For this review, take the finished solid that the model builds, in its own axes (mm). A direction names the side the tool comes from. Give positions to 0.01 mm unless a question says otherwise; leave off trailing zeros. Order: outer loops, then holes, each group sorted by start corner. A loop starts at its lowest first (then second) coordinate and runs counter-clockwise, first axis right, second up. Notation, with made-up numbers: M -26,45 L -15,45 A19 ccw -15,52 Z; hole C 28,-4 d8. An arc over 180 degrees is marked long. Use CSV: the item, a comma, the result in double quotes. Start each with the question number.
(1) Clearance check with flat-ended pins moving along their axes: P1, Ø4, axis at x = 32, y = -44.5, coming from the -Z side; P2, Ø1.2, axis at y = 33, z = 2, coming from the +X side. State where each tip first meets the part, or that it passes through.
(2) Consider section C-C (x = 31). Write out the cut boundary in (y, z).
(3) Draft analysis for pull direction X (two halves, no side actions). For faces 1 (the face through (60, -60, 2)), 2 (the face through (0.752, 39.287, 1.972)), 3 (the face through (11.4, 32.19, 1.97)), state which applies: pulls with the +X half, pulls with the -X half, needs draft (parallel to the pull), parting line crosses it, or undercut.
(4) Consider section D-D (z = 1.25). Give the number of separate pieces and of enclosed holes in the cut face, and give its area (3 significant figures).
(5) Consider section B-B (y = 10). Write out the cut boundary in (x, z), and give its area (3 significant figures).
(6) Wall thickness on L1, parallel to Y at x = 70, z = 2.75; L2, parallel to Y at x = 50.5, z = 1.15; L3, parallel to Y at x = 30, z = 2: over which ranges is each line inside the solid? List them lowest first. Write a range as from..to.
(7) Tool access review of faces 4 (the face through (60, 0, 2)), 5 (the face through (9.44, 7.46, 1.97)): name each direction out of +Z, -Z, +X, -X, +Y, -Y from which nothing blocks a thin tool from reaching the whole face with its end or side.
(8) Consider section A-A (x = 70). Write out the cut boundary in (y, z).
```python
from build123d import *

# Parameters (mm, degrees)
SKETCH_1_R      = 2.6
EXTRUDE_1_DEPTH = 4


with BuildPart() as part:
    # Эскиз1 → Бобышка-Вытянуть1 (new body)
    with BuildSketch(Plane.XY):
        with BuildLine():
            Line((40.732233047, -79.267766953), (79.267766953, -40.732233047))
            ThreePointArc((79.267766953, -40.732233047), (79.809698831, -39.921174675), (80, -38.964466094))
            Line((80, -38.964466094), (80, -2.5))
            ThreePointArc((80, -2.5), (79.267766953, -0.732233047), (77.5, 0))
            Line((77.5, 0), (41.035533906, 0))
            ThreePointArc((41.035533906, 0), (40.078825325, 0.190301169), (39.267766953, 0.732233047))
            Line((39.267766953, 0.732233047), (20.732233047, 19.267766953))
            ThreePointArc((20.732233047, 19.267766953), (20.190301169, 20.078825325), (20, 21.035533906))
            Line((20, 21.035533906), (20, 37.5))
            ThreePointArc((20, 37.5), (19.267766953, 39.267766953), (17.5, 40))
            Line((17.5, 40), (2.5, 40))
            ThreePointArc((2.5, 40), (0.732233047, 39.267766953), (0, 37.5))
            Line((0, 37.5), (0, 0))
            Line((0, 0), (0, -77.5))
            ThreePointArc((0, -77.5), (0.732233047, -79.267766953), (2.5, -80))
            Line((2.5, -80), (38.964466094, -80))
            ThreePointArc((38.964466094, -80), (39.921174675, -79.809698831), (40.732233047, -79.267766953))
        make_face()
        with Locations((10, -10)):
            Circle(SKETCH_1_R, mode=Mode.SUBTRACT)
        with Locations((30, -10)):
            Circle(SKETCH_1_R, mode=Mode.SUBTRACT)
        with Locations((30, -30)):
            Circle(SKETCH_1_R, mode=Mode.SUBTRACT)
        with Locations((30, -50)):
            Circle(SKETCH_1_R, mode=Mode.SUBTRACT)
        with Locations((30, -70)):
            Circle(SKETCH_1_R, mode=Mode.SUBTRACT)
        with Locations((10, -30)):
            Circle(SKETCH_1_R, mode=Mode.SUBTRACT)
        with Locations((10, -50)):
            Circle(SKETCH_1_R, mode=Mode.SUBTRACT)
        with Locations((10, -70)):
            Circle(SKETCH_1_R, mode=Mode.SUBTRACT)
        with Locations((50, -10)):
            Circle(SKETCH_1_R, mode=Mode.SUBTRACT)
        with Locations((50, -30)):
            Circle(SKETCH_1_R, mode=Mode.SUBTRACT)
        with Locations((70, -10)):
            Circle(SKETCH_1_R, mode=Mode.SUBTRACT)
        with Locations((70, -30)):
            Circle(SKETCH_1_R, mode=Mode.SUBTRACT)
        with Locations((10, 10)):
            Circle(SKETCH_1_R, mode=Mode.SUBTRACT)
        with Locations((10, 30)):
            Circle(SKETCH_1_R, mode=Mode.SUBTRACT)
    extrude(amount=EXTRUDE_1_DEPTH)


solid = part.part
```
Check result:
1,P1,"stops at z = 0"
1,P2,"stops at x = 20"
2,outline,"M -80,0 L -72.4,0 L -72.4,4 L -80,4 Z; M -67.6,0 L -52.4,0 L -52.4,4 L -67.6,4 Z; M -47.6,0 L -32.4,0 L -32.4,4 L -47.6,4 Z; M -27.6,0 L -12.4,0 L -12.4,4 L -27.6,4 Z; M -7.6,0 L 9,0 L 9,4 L -7.6,4 Z"
3,face 1,"pulls with the +X half"
3,face 2,"pulls with the -X half"
3,face 3,"undercut"
4,separate pieces,"1"
4,enclosed holes,"14"
4,area,"6,300 mm^2"
5,outline,"M 0,0 L 7.4,0 L 7.4,4 L 0,4 Z; M 12.6,0 L 30,0 L 30,4 L 12.6,4 Z"
5,area,"99.2 mm^2"
6,L1,"y = -50..-32.6, -27.4..-12.6, -7.4..0"
6,L2,"y = -69.5..-32.55, -27.45..-12.55, -7.45..0"
6,L3,"y = -80..-72.6, -67.4..-52.6, -47.4..-32.6, -27.4..-12.6, -7.4..10"
7,face 4,"+Z, -Z, +X, +Y"
7,face 5,"+Z, -Z"
8,outline,"M -50,0 L -32.6,0 L -32.6,4 L -50,4 Z; M -27.4,0 L -12.6,0 L -12.6,4 L -27.4,4 Z; M -7.4,0 L 0,0 L 0,4 L -7.4,4 Z"
